CAD build for the part. Positions are in the model's coordinates, mm. Round coordinates to 2 decimals unless told otherwise and drop trailing zeros. Write each loop counter-clockwise with the first axis right and the second up, starting at its lowest first coordinate (ties: lowest second). Pieces come first, ordered by that corner, then holes. Notation, with made-up numbers: (-31.5, -22.5) - (-7.5, -22.5) arc R30 ccw to (-7.5, 15.5) - close; hole circle Ø5 at (10.5, 74). An arc over 180 degrees is marked (long way). Answer in a Markdown table with one row per item.
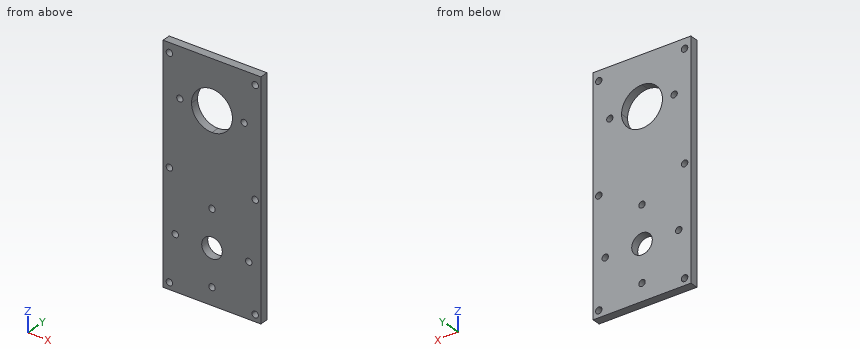
```python
from build123d import *

# Parameters (mm, degrees)
SKETCH1_R           = 1.25
SKETCH1_R_2         = 1.22
SKETCH1_R_3         = 4
BOSS_EXTRUDE1_DEPTH = 3.175


with BuildPart() as part:
    # Sketch1 → Boss-Extrude1 (new body)
    with BuildSketch(Plane(origin=(0, 0, 0), x_dir=(1, 0, 0), z_dir=(0, 1, 0))):
        Polygon((-19, 71), (-19, -19), (0, -19), (19, -19), (19, 71), align=None)
        with Locations(Location((-16.556995364, -15.248859434, 0), (0, 0, 270))):
            Circle(SKETCH1_R, mode=Mode.SUBTRACT)
        with Locations(Location((-12.5, 0, 0), (0, 0, 270))):
            Circle(SKETCH1_R_2, mode=Mode.SUBTRACT)
        with BuildLine():
            ThreePointArc((7.9375, 0), (5.612660076, -5.612660076), (0, -7.9375))
            ThreePointArc((0, -7.9375), (-5.612660076, -5.612660076), (-7.9375, 0))
            ThreePointArc((-7.9375, 0), (-5.612660076, 5.612660076), (0, 7.9375))
            ThreePointArc((0, 7.9375), (5.612660076, 5.612660076), (7.9375, 0))
        make_face(mode=Mode.SUBTRACT)
        with Locations(Location((16.785315207, -15.248859434, 0), (0, 0, 270))):
            Circle(SKETCH1_R, mode=Mode.SUBTRACT)
        with Locations(Location((12.5, 0, 0), (0, 0, 270))):
            Circle(SKETCH1_R_2, mode=Mode.SUBTRACT)
        with BuildLine():
            ThreePointArc((-16.556995364, 25.292624917), (-17.806995364, 26.542624917), (-16.556995364, 27.792624917))
            ThreePointArc((-16.556995364, 27.792624917), (-15.306995364, 26.542624917), (-16.556995364, 25.292624917))
        make_face(mode=Mode.SUBTRACT)
        with Locations(Location((-14.2875, 50, 0), (0, 0, 270))):
            Circle(SKETCH1_R, mode=Mode.SUBTRACT)
        with BuildLine():
            ThreePointArc((-16.556995364, 67.084109267), (-17.440878841, 69.217992744), (-15.306995364, 68.334109267))
            ThreePointArc((-15.306995364, 68.334109267), (-15.673111888, 67.450225791), (-16.556995364, 67.084109267))
        make_face(mode=Mode.SUBTRACT)
        with BuildLine():
            ThreePointArc((16.785315207, 25.292624917), (15.535315207, 26.542624917), (16.785315207, 27.792624917))
            ThreePointArc((16.785315207, 27.792624917), (18.035315207, 26.542624917), (16.785315207, 25.292624917))
        make_face(mode=Mode.SUBTRACT)
        with Locations(Location((0, 35.7125, 0), (0, 0, 270))):
            Circle(SKETCH1_R, mode=Mode.SUBTRACT)
        with Locations(Location((14.2875, 50, 0), (0, 0, 270))):
            Circle(SKETCH1_R, mode=Mode.SUBTRACT)
        with Locations(Location((0, 64.2875, 0), (0, 0, 270))):
            Circle(SKETCH1_R, mode=Mode.SUBTRACT)
        with Locations(Location((0, 50, 0), (0, 0, 270))):
            Circle(SKETCH1_R_3, mode=Mode.SUBTRACT)
        with BuildLine():
            ThreePointArc((16.785315207, 67.084109267), (15.90143173, 67.450225791), (15.535315207, 68.334109267))
            ThreePointArc((15.535315207, 68.334109267), (17.669198683, 69.217992744), (16.785315207, 67.084109267))
        make_face(mode=Mode.SUBTRACT)
    extrude(amount=BOSS_EXTRUDE1_DEPTH)


solid = part.part
```
Q1. Saw through at B-B on y = 1.5. Count the separate pieces of the cut face and the enclosed holes in it, then the cut area to 3 significant figures.
Computed:
| item | result |
|---|---|
| separate pieces | 1 |
| enclosed holes | 14 |
| area | 3,110 mm2 |
Q2. Saw through at C-C on z = -64. List the corners of the cut face in (x, y) (3 decimals).
Computed:
| item | result |
|---|---|
| outline | (-19, 0) - (-1.216, 0) - (-1.216, 3.175) - (-19, 3.175) - close; (1.216, 0) - (19, 0) - (19, 3.175) - (1.216, 3.175) - close |
Q3. Saw through at A-A on z = -50. List the corners of the cut face in (x, y) (1 decimal), then the cut area to 3 significant figures.
Computed:
| item | result |
|---|---|
| outline | (-19, 0) - (-15.5, 0) - (-15.5, 3.2) - (-19, 3.2) - close; (-13, 0) - (-4, 0) - (-4, 3.2) - (-13, 3.2) - close; (4, 0) - (13, 0) - (13, 3.2) - (4, 3.2) - close; (15.5, 0) - (19, 0) - (19, 3.2) - (15.5, 3.2) - close |
| area | 79.4 mm2 |
Q4. Drill centre lines: line 1 (X direction, y = 2.35, z = -50); line 2 (Z direction, x = 13.5, y = 2.75); line 3 (Z direction, x = -1.5, y = 0.4). Where is each one in solid material? Low to high.
Computed:
| item | result |
|---|---|
| line 1 | x = -19 to -15.54, -13.04 to -4, 4 to 13.04, 15.54 to 19 |
| line 2 | z = -71 to -50.97, -49.03 to -0.7, 0.7 to 19 |
| line 3 | z = -71 to -53.71, -46.29 to -7.79, 7.79 to 19 |
Q5. Flat gauge pin, fed straight in: pin 1 (2 mm diameter, centred on x = -16.56, z = 15.25, fed in from +Y). Where does the tip first touch, or does it go through?
Computed:
| item | result |
|---|---|
| pin 1 | passes through |
